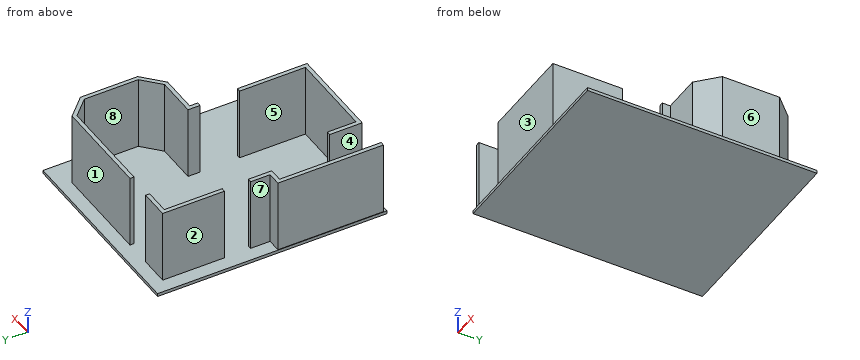
```python
from build123d import *

# Parameters (mm, degrees)
SKETCH001_W  = 249.235731
SKETCH001_H  = 289.366922
PAD_DEPTH    = 4
PAD001_DEPTH = 93


with BuildPart() as part:
    # Sketch001 → Pad (new body)
    with BuildSketch(Plane.XY):
        with Locations((101.953362, -122.984355)):
            Rectangle(SKETCH001_W, SKETCH001_H)
    extrude(amount=PAD_DEPTH)

    # Sketch (on Face6 of Pad) → Pad001 (join)
    with BuildSketch(Plane.XY.offset(4)):
        Polygon((-17, -135.5), (0, -135.5), (0, -106), (-5, -106), (-5, -130.5), (-22, -130.5), (-22, -263.55), (-17, -263.55), align=None)
        Polygon((0, 0), (32, 0), (32, 5), (-5, 5), (-5, -73), (0, -73), align=None)
        Polygon((66, 5), (66, 0), (190, 0), (211.023543, -21.401183), (211.023543, -89.401183), (189.213253, -110), (138.213253, -110), (138.213253, -125), (143.213253, -125), (143.213253, -115), (191.201161, -115), (216.023543, -91.5564), (216.023543, -19.356138), (192.097187, 5), align=None)
        Polygon((138.2, -257.999998), (28.2, -257.999998), (28.2, -221.999998), (23.2, -221.999998), (23.2, -262.999998), (143.2, -262.999998), (143.2, -174.999998), (138.2, -174.999998), align=None)
    extrude(amount=PAD001_DEPTH)


solid = part.part
```
Check sheet for the modelled part. Datum: model origin and axes. Units: mm. Face numbers are marked on the shaded views. A direction names the side the tool comes from. Round coordinates to 2 decimals unless told otherwise and drop trailing zeros. Write each loop counter-clockwise with the first axis right and the second up, starting at its lowest first coordinate (ties: lowest second). Pieces come first, ordered by that corner, then holes. Notation, with made-up numbers: (47.5, -27) -> (52.5, -27) arc R16 cw to (52.5, -6) -> close; hole circle Ø6 at (44, 60.5). An arc over 180 degrees is marked (long way). Put each result on its own line as item: value.
(1) Sectioned sample at D-D (y = -29). Enter the section's corners in (x, z), plus the area to 3 significant figures.
Values found:
outline: (-22.66, 0) -> (226.57, 0) -> (226.57, 4) -> (216.02, 4) -> (216.02, 97) -> (211.02, 97) -> (211.02, 4) -> (0, 4) -> (0, 97) -> (-5, 97) -> (-5, 4) -> (-22.66, 4) -> close
area: 1,930 mm^2
(2) Sectioned sample at B-B (y = -245.5). Enter the section's corners in (x, z).
Values found:
outline: (-22.66, 0) -> (226.57, 0) -> (226.57, 4) -> (143.2, 4) -> (143.2, 97) -> (138.2, 97) -> (138.2, 4) -> (28.2, 4) -> (28.2, 97) -> (23.2, 97) -> (23.2, 4) -> (-17, 4) -> (-17, 97) -> (-22, 97) -> (-22, 4) -> (-22.66, 4) -> close
(3) Sectioned sample at A-A (x = 5). Enter the section's corners in (y, z), plus the area to 3 significant figures.
Values found:
outline: (-267.67, 0) -> (21.7, 0) -> (21.7, 4) -> (5, 4) -> (5, 97) -> (0, 97) -> (0, 4) -> (-267.67, 4) -> close
area: 1,620 mm^2
(4) Material ranges on line 1 (X direction, y = -249, z = 45.5); line 2 (X direction, y = -31, z = 49); line 3 (Y direction, x = 158, z = 60.5), recorded low to high.
Values found:
line 1: x = -22 to -17, 23.2 to 28.2, 138.2 to 143.2
line 2: x = -5 to 0, 211.02 to 216.02
line 3: y = -115 to -110, 0 to 5
(5) Sectioned sample at C-C (z = 69.5). Count the separate pieces of the cut face and the enclosed holes in it, plus the area to 3 significant figures.
Values found:
separate pieces: 4
enclosed holes: 0
area: 4,220 mm^2
(6) Go/stop test with flat-tipped pins: pin 1 Ø5.5 at (x, z) = (26.5, 51) entering from +Y; pin 2 Ø25 at (y, z) = (-217.5, 62.5) entering from -X; pin 3 Ø4 at (x, y) = (169, -75) entering from +Z; pin 4 Ø8 at (x, y) = (77, -173.5) entering from -Z. Record where each tip stops, or that it passes through.
Values found:
pin 1: stops at y = 5
pin 2: stops at x = -22
pin 3: stops at z = 4
pin 4: stops at z = 0
(7) Tool access check on the marked faces 1, 2, 3, 4 and 5. Record the directions out of +Z, -Z, +X, -X, +Y, -Y that give a thin tool (end or side, any length) a straight path to the whole face; none if there is none.
Values found:
face 1: +Z, +X, -X, +Y
face 2: +Z, -X, +Y
face 3: +Z, +X, -Y
face 4: +Z, -Y
face 5: +Z
(8) Mould release check, pull along X, two halves, no side actions. Record for the marked faces 6, 7 and 8: released by +X, released by -X, zero draft, split by the parting line, or undercut.
Values found:
face 6: released by +X
face 7: released by -X
face 8: undercut
